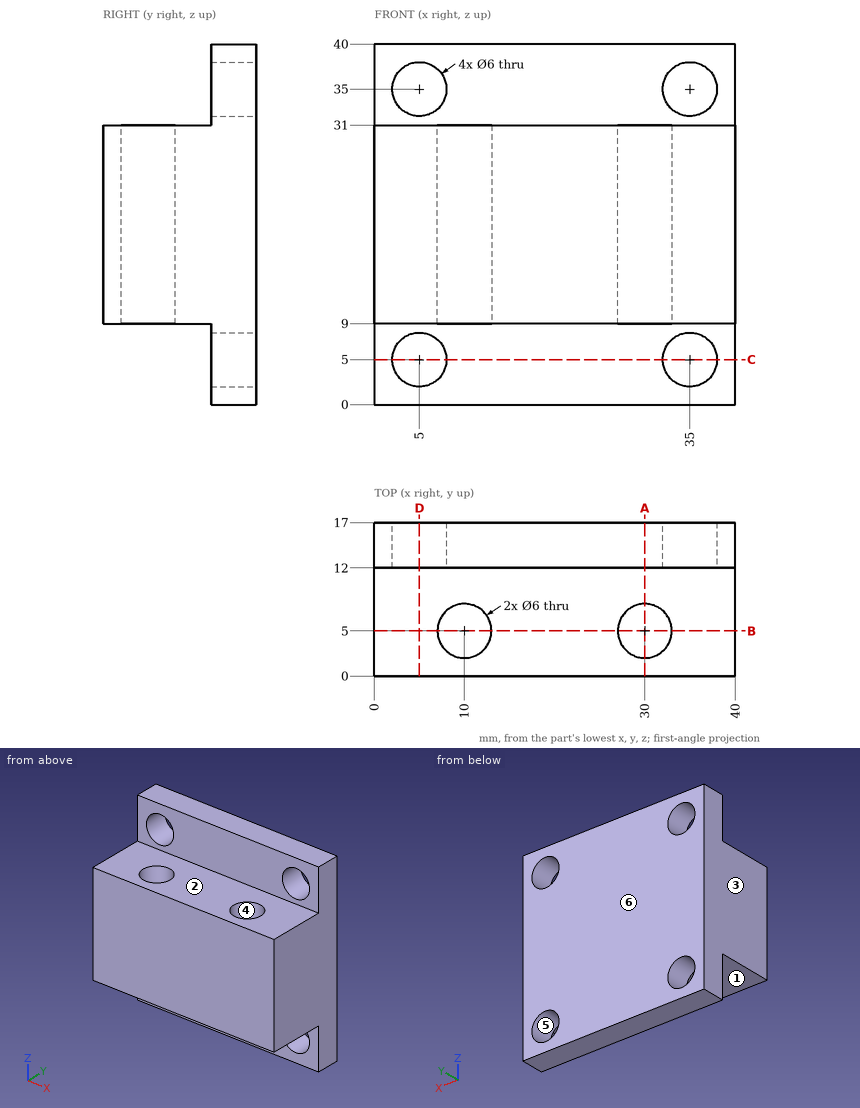
Check sheet for the drawn part. Datum: minimum x, y, z corner. Units: mm. A direction names the side the tool comes from. Round coordinates to 2 decimals unless told otherwise and drop trailing zeros. Order: outer loops, then holes, each group sorted by start corner. A loop starts at its lowest first (then second) coordinate and runs counter-clockwise, first axis right, second up. Notation, with made-up numbers: (52.5, 86) - (104.5, 86) arc R26 cw to (104.5, 123) - close; hole circle Ø2 at (74.25, 72). An arc over 180 degrees is marked (long way). Use a Markdown table: item, result. Add a question column.
(1) Depth check by flat-ended pin: pin 1 (6 mm diameter, centred on x = 8, z = 28.5, fed in from -Y); pin 2 (7 mm diameter, centred on x = 30, y = 5, fed in from +Z); pin 3 (4 mm diameter, centred on x = 23, z = 35, fed in from -Y); pin 4 (9.5 mm diameter, centred on x = 22.5, y = 4.5, fed in from -Z). Enter the tip coordinate at first touch or a pass-through.
(2) Sectioned sample at A-A, the plane x = 30. Enter the section's corners in (y, z), and give its area (3 significant figures).
(3) Release check for a two-part mould opening along Y. For the marked faces 4, 5 and 6 record: pulls with the +Y half, pulls with the -Y half, needs draft (parallel to the pull), parting line crosses it, or undercut.
(4) Sectioned sample at D-D, the plane x = 5. Enter the section's corners in (y, z).
(5) Sectioned sample at B-B, the plane y = 5. Enter the section's corners in (x, z), and give its area (3 significant figures).
(6) Tool access check on the marked faces 1, 2 and 3. Record the directions out of +Z, -Z, +X, -X, +Y, -Y that give a thin tool (end or side, any length) a straight path to the whole face; none if there is none.
(7) Sectioned sample at C-C, the plane z = 5. Enter the section's corners in (x, y).
(8) Material ranges on line 1 along Z through (x, y) = (5, 15.95); line 2 along X through (y, z) = (4.75, 13), recorded low to high. Write a range as [from, to].
Answers below:
| question | item | result |
|---|---|---|
| 1 | pin 1 | y = 0 |
| 1 | pin 2 | z = 31 |
| 1 | pin 3 | y = 12 |
| 1 | pin 4 | z = 9 |
| 2 | outline | (0, 9) - (2, 9) - (2, 31) - (0, 31) - close; (8, 9) - (12, 9) - (12, 0) - (17, 0) - (17, 40) - (12, 40) - (12, 31) - (8, 31) - close |
| 2 | area | 332 mm² |
| 3 | face 4 | undercut |
| 3 | face 5 | needs draft |
| 3 | face 6 | pulls with the +Y half |
| 4 | outline | (0, 9) - (12, 9) - (12, 8) - (17, 8) - (17, 32) - (12, 32) - (12, 31) - (0, 31) - close; (12, 0) - (17, 0) - (17, 2) - (12, 2) - close; (12, 38) - (17, 38) - (17, 40) - (12, 40) - close |
| 5 | outline | (0, 9) - (7, 9) - (7, 31) - (0, 31) - close; (13, 9) - (27, 9) - (27, 31) - (13, 31) - close; (33, 9) - (40, 9) - (40, 31) - (33, 31) - close |
| 5 | area | 616 mm² |
| 6 | face 1 | -Z, +X, -X, -Y |
| 6 | face 2 | +Z, +X, -X, -Y |
| 6 | face 3 | +Z, -Z, -X, +Y, -Y |
| 7 | outline | (0, 12) - (2, 12) - (2, 17) - (0, 17) - close; (8, 12) - (32, 12) - (32, 17) - (8, 17) - close; (38, 12) - (40, 12) - (40, 17) - (38, 17) - close |
| 8 | line 1 | [0, 2], [8, 32], [38, 40] |
| 8 | line 2 | [0, 7.01], [12.99, 27.01], [32.99, 40] |
